Answer from the drawing. Dimensions are ordinates in mm from the lowest x, y and z of the part. Coordinates: 2 decimals unless noted, no trailing zeros. Order: outer loops, then holes, each group sorted by start corner. A loop starts at its lowest first (then second) coordinate and runs counter-clockwise, first axis right, second up. Notation, with made-up numbers: M -14,18.5 L -6,18.5 A8 cw -6,25.5 Z; hole C -21,-29.5 d5. An arc over 180 degrees is marked long. Write each question's results on one line, items separated by ' | '.
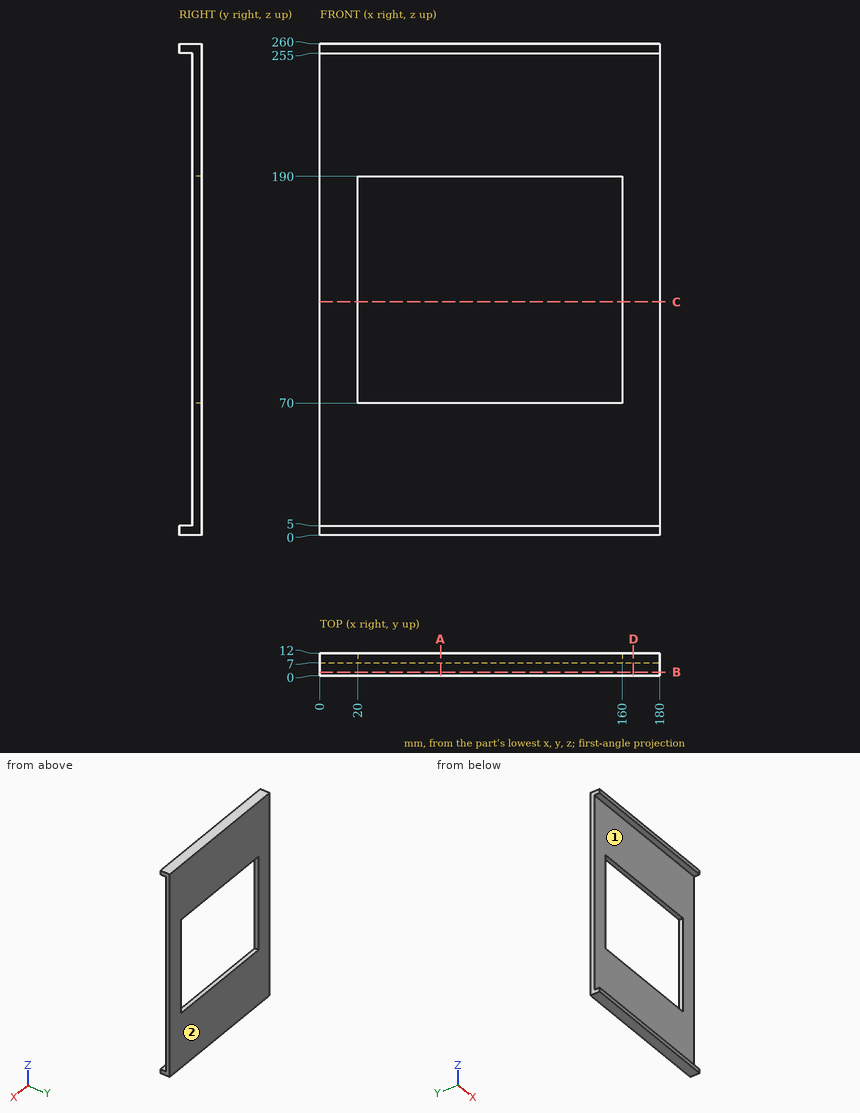
(1) The part is cut by section D-D, the plane x = 166. Write down the section's boundary in (y, z).
Conclusion:
outline: M 0,0 L 12,0 L 12,260 L 0,260 L 0,255 L 7,255 L 7,5 L 0,5 Z
(2) The mould has two halves that part along Z. Classify the marked faces 1 and 2: pulls with the +Z half, pulls with the -Z half, needs draft (parallel to the pull), parting line crosses it, or undercut.
Conclusion:
face 1: undercut | face 2: needs draft
(3) Straight lines are drawn through the part: line 1 (Z direction, x = 39.5, y = 9); line 2 (X direction, y = 8.5, z = 73); line 3 (Z direction, x = 109.5, y = 1.25). For each, find the intervals that lie inside material, in ascending order.
Conclusion:
line 1: 0 to 70, 190 to 260 | line 2: 0 to 20, 160 to 180 | line 3: 0 to 5, 255 to 260
(4) The part is cut by section B-B, the plane y = 2. Write down the section's boundary in (x, z), then the cut area to 3 significant figures.
Conclusion:
outline: M 0,0 L 180,0 L 180,5 L 0,5 Z; M 0,255 L 180,255 L 180,260 L 0,260 Z | area: 1,800 mm²
(5) The part is cut by section C-C, the plane z = 123.5. Write down the section's boundary in (x, y), then the cut area to 3 significant figures.
Conclusion:
outline: M 0,7 L 20,7 L 20,12 L 0,12 Z; M 160,7 L 180,7 L 180,12 L 160,12 Z | area: 200 mm²
(6) The part is cut by section A-A, the plane x = 64. Write down the section's boundary in (y, z).
Conclusion:
outline: M 0,0 L 12,0 L 12,70 L 7,70 L 7,5 L 0,5 Z; M 0,255 L 7,255 L 7,190 L 12,190 L 12,260 L 0,260 Z
